from build123d import *

# Parameters (mm, degrees)
SKETCH1_W           = 60
SKETCH1_H           = 60
SKETCH1_R           = 1.5
BOSS_EXTRUDE1_DEPTH = 3
BOSS_EXTRUDE2_DEPTH = 22


with BuildPart() as part:
    # Sketch1 → Boss-Extrude1 (new body)
    with BuildSketch(Plane(origin=(0, 0, 0), x_dir=(1, 0, 0), z_dir=(0, 1, 0))):
        with Locations((30, 30)):
            Rectangle(SKETCH1_W, SKETCH1_H)
        with Locations((3.5, 3.5)):
            Circle(SKETCH1_R, mode=Mode.SUBTRACT)
        with Locations((56.5, 3.5)):
            Circle(SKETCH1_R, mode=Mode.SUBTRACT)
        with Locations((56.5, 56.5)):
            Circle(SKETCH1_R, mode=Mode.SUBTRACT)
        with Locations((3.5, 56.5)):
            Circle(SKETCH1_R, mode=Mode.SUBTRACT)
    extrude(amount=BOSS_EXTRUDE1_DEPTH)

    # Sketch2 → Boss-Extrude2 (add)
    with BuildSketch(Plane(origin=(0, 3, 0), x_dir=(1, 0, 0), z_dir=(0, 1, 0))):
        Polygon((7, 60), (53, 60), (53, 53), (60, 53), (60, 7), (53, 7), (53, 0), (7, 0), (7, 7), (0, 7), (0, 53), (7, 53), align=None)
    extrude(amount=BOSS_EXTRUDE2_DEPTH)


solid = part.part
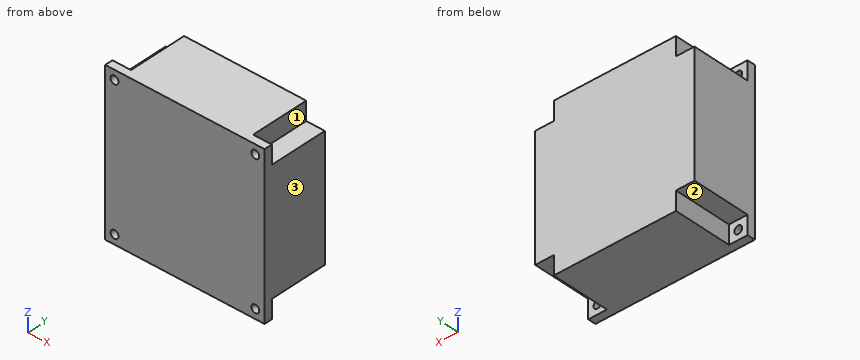
Can you work these out from the model? Positions are in its coordinate system, mm. Face numbers are marked on the shaded views. A direction names the side the tool comes from. Round coordinates to 2 decimals unless told otherwise and drop trailing zeros. Write each loop counter-clockwise with the first axis right and the second up, starting at its lowest first coordinate (ties: lowest second). Pieces come first, ordered by that corner, then holes. Notation, with made-up numbers: (-27, 63.5) -> (24, 63.5) arc R30 cw to (24, 99.5) -> close; hole circle Ø9 at (67, 76). An arc over 180 degrees is marked (long way). Use one line per item in the form item = value. Start each with the question number.
Q1. Imagine slicing it at B-B (x = 3.5). Please give me the cut outline in (y, z).
Q2. Imagine slicing it at A-A (z = -3.5). Please give me the cut outline in (x, y).
Q3. I'm going to push flat-ended pins straight in: P1, Ø2, axis at y = 10.5, z = -3.5, coming from the +X side; P2, Ø3.5, axis at x = 2.5, y = 11.5, coming from the -Z side; P3, Ø2, axis at x = 56, y = 14.5, coming from the +Z side. Where does each tip first touch, or does it pass through?
Q4. If I drill on probe 1 along Z at (x, y) = (56.5, 0.85); probe 2 along X at (y, z) = (1.3, -3.5); probe 3 along X at (y, z) = (11.5, -53.5), over which ranges is the centre line in solid material (lowest first)? Write a range as [from, to].
Q5. Imagine slicing it at C-C (y = 13.75). Please give me the cut outline in (x, z), then the cut area to 3 significant figures.
Q6. Which directions (+Z, -Z, +X, -X, +Y, -Y) give clear straight access to the entire face, cutting with the end or side of a thin tool? Please do the marked faces 1, 2 and 3.
Worked out:
q1.outline = (0, -60) -> (3, -60) -> (3, -58) -> (0, -58) -> close; (0, -55) -> (3, -55) -> (3, -53) -> (25, -53) -> (25, -7) -> (3, -7) -> (3, -5) -> (0, -5) -> close; (0, -2) -> (3, -2) -> (3, 0) -> (0, 0) -> close
q2.outline = (0, 0) -> (2, 0) -> (2, 3) -> (0, 3) -> close; (5, 0) -> (55, 0) -> (55, 3) -> (53, 3) -> (53, 25) -> (7, 25) -> (7, 3) -> (5, 3) -> close; (58, 0) -> (60, 0) -> (60, 3) -> (58, 3) -> close
q3.P1 = 53
q3.P2 = -53
q3.P3 = -7
q4.probe_1 = [-60, -58], [-55, -5], [-2, 0]
q4.probe_2 = [0, 2], [5, 55], [58, 60]
q4.probe_3 = [7, 53]
q5.outline = (0, -53) -> (7, -53) -> (7, -60) -> (53, -60) -> (53, -53) -> (60, -53) -> (60, -7) -> (53, -7) -> (53, 0) -> (7, 0) -> (7, -7) -> (0, -7) -> close
q5.area = 3,400 mm^2
q6.face_1 = +Z, +X, +Y
q6.face_2 = -Z, -X, +Y
q6.face_3 = +Z, -Z, +X, +Y, -Y
